Solid Edge part; units mm, degrees
sketch "Sketch1" plane through (0, 0, 0) normal (1, 0, 0) x (0, 1, 0)
  line L0 (74, 81.0476) -> (74, 0)
  line L1 (44, 80) -> (74, 81.0476)
  line L2 (44, 80) -> (44, 44.0365)
  line L3 (0, 42.5) -> (44, 44.0365)
  line L4 (0, 42.5) -> (0, 0)
  dimension "D1" = 44
  dimension "D2" = 74
revolve "RevolvedProtrusion1" add sketch "Sketch1" angle 360 about axis through (0, 0, 0) along (0, 1, 0)
sketch "Sketch2" plane through (0, 0, 0) normal (0, -1, 0) x (1, 0, 0)
  circle A0 centre (0, 0) radius 28
extrude "Cutout1" cut sketch "Sketch2" against normal blind 250.3843
fillet "Raccordi" radius 6 3 edges at (0, 0, 42.5) (0, 44, 44.0365) (0, 44, 80)
properties material "Acciaio"
Design review of the part built by this model. Coordinates are the model's own, in mm. A direction names the side the tool comes from. Give positions to 0.01 mm unless a question says otherwise; leave off trailing zeros. Order: outer loops, then holes, each group sorted by start corner. A loop starts at its lowest first (then second) coordinate and runs counter-clockwise, first axis right, second up. Notation, with made-up numbers: (33, 57.5) - (54, 57.5) arc R19 cw to (54, 77.5) - close; hole circle Ø10 at (22.25, -6.75). An arc over 180 degrees is marked (long way). Write item = value, one per line. Start each with the question number.
Q1. Clearance check with flat-ended pins moving along their axes: pin 1 Ø8 at (x, y) = (21, 40.5) entering from -Z; pin 2 Ø4 at (y, z) = (66.5, 8.5) entering from +X; pin 3 Ø4 at (y, z) = (39, -17.5) entering from +X. State where each tip first meets the part, or that it passes through.
Q2. Mouldability with a two-part tool opening along Z and no side actions: class faces 1 (the face through (-49.01, 59.37, -63.91)), 2 (the face through (25.865, 36.482, -10.724)), 3 (the face through (1, 74, 35)) as released by +Z, released by -Z, zero draft, split by the parting line, or undercut.
Q3. We need section B-B on x = 0. State the section outline as (y, z) points.
Q4. We need section C-C on y = 10.5. State the section outline as (x, z) points, plus the area to 3 significant figures.
Q5. Tool access review of faces 4 (the face through (-15, 44, 48)), 5 (the face through (-27, 0, -8)): name each direction out of +Z, -Z, +X, -X, +Y, -Y from which nothing blocks a thin tool from reaching the whole face with its end or side.
Q6. We need section D-D on y = 41. State the section outline as (x, z) points, plus the area to 3 significant figures.
Q7. We need section A-A on z = 0. State the section outline as (x, y) points, plus the area to 3 significant figures.
Q8. To check wall thickness, follow L1, parallel to Z at x = -10, y = 26; L2, parallel to Z at x = 0, y = 51; L3, parallel to X at y = 69, z = 3.5. State the ranges of each line that lie inside material, in increasing order. Write a range as from..to.
Working result:
q1.pin_1 = -73.73
q1.pin_2 = 80.54
q1.pin_3 = 41.32
q2.face_1 = split by the parting line
q2.face_2 = undercut
q2.face_3 = zero draft
q3.outline = (0, -36.71) arc R6 ccw to (5.79, -42.7) - (38.21, -43.83) arc R6 cw to (44, -49.83) - (44, -74.21) arc R6 ccw to (49.79, -80.2) - (74, -81.05) - (74, -28) - (0, -28) - close; (0, 28) - (74, 28) - (74, 81.05) - (49.79, 80.2) arc R6 ccw to (44, 74.21) - (44, 49.83) arc R6 cw to (38.21, 43.83) - (5.79, 42.7) arc R6 ccw to (0, 36.71) - close
q4.outline = circle Ø85.73 at (0, 0); hole circle Ø56 at (0, 0)
q4.area = 3,310 mm²
q5.face_4 = -Y
q5.face_5 = +Z, -Z, +X, -X, -Y
q6.outline = circle Ø89.27 at (0, 0); hole circle Ø56 at (0, 0)
q6.area = 3,800 mm²
q7.outline = (-81.05, 74) - (-80.2, 49.79) arc R6 ccw to (-74.21, 44) - (-49.83, 44) arc R6 cw to (-43.83, 38.21) - (-42.7, 5.79) arc R6 ccw to (-36.71, 0) - (-28, 0) - (-28, 74) - close; (28, 0) - (36.71, 0) arc R6 ccw to (42.7, 5.79) - (43.83, 38.21) arc R6 cw to (49.83, 44) - (74.21, 44) arc R6 ccw to (80.2, 49.79) - (81.05, 74) - (28, 74) - close
q7.area = 4,480 mm²
q8.L1 = -42.24..-26.15, 26.15..42.24
q8.L2 = -80.24..-28, 28..80.24
q8.L3 = -80.8..-27.78, 27.78..80.8
